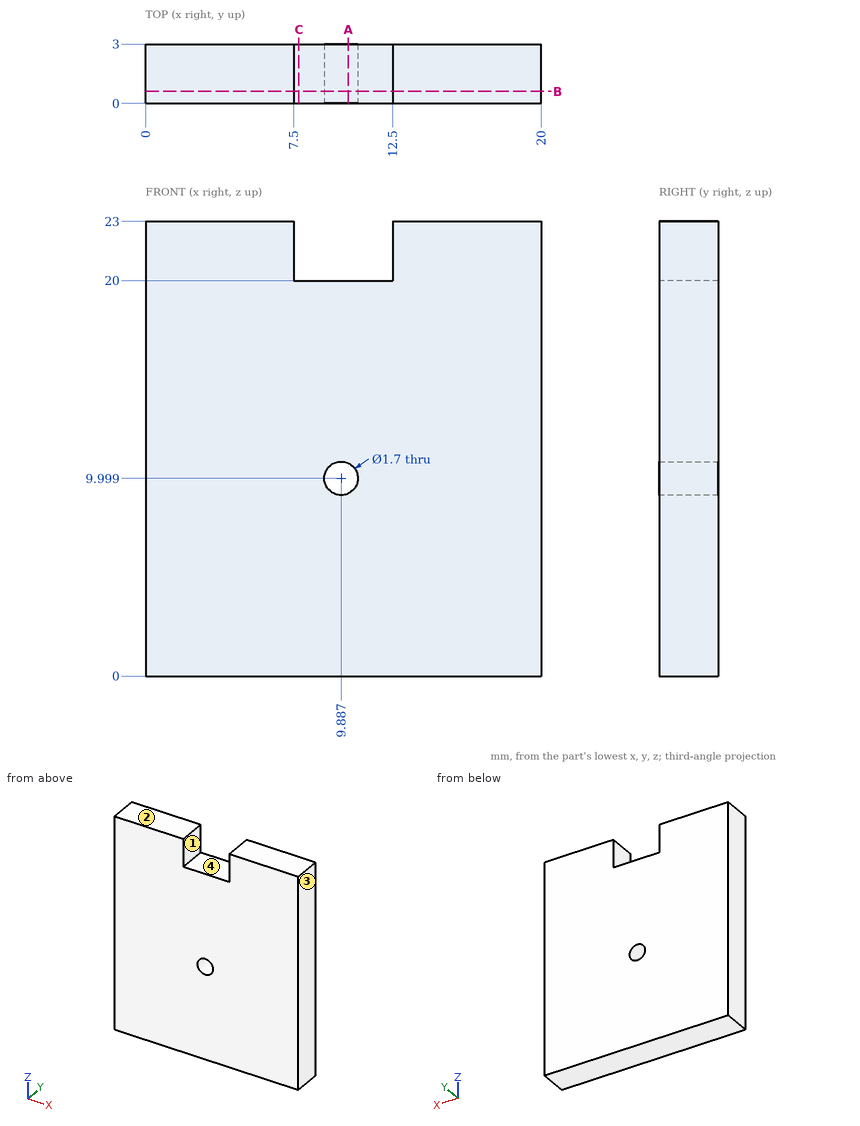
Drawing for the job (mm, zero at the part's lowest x, y, z). Give positions to 0.01 mm unless a question says otherwise; leave off trailing zeros. Order: outer loops, then holes, each group sorted by start corner. A loop starts at its lowest first (then second) coordinate and runs counter-clockwise, first axis right, second up. Notation, with made-up numbers: (-25.75, 61.5) - (31.25, 61.5) arc R16 ccw to (31.25, 83.5) - close; hole circle Ø4 at (29, -10.75). An arc over 180 degrees is marked (long way). Use one line per item in the form item = value.
Item 1: Slice it at B-B on y = 0.6. Give the cut face in (x, z).
Solution:
outline = (0, 0) - (20, 0) - (20, 23) - (12.5, 23) - (12.5, 20) - (7.5, 20) - (7.5, 23) - (0, 23) - close; hole circle Ø1.7 at (9.89, 10)
Item 2: Pin check, flat tips, straight feed: pin 1 Ø1 at (x, z) = (9.89, 10) entering from +Y; pin 2 Ø1.5 at (x, y) = (9, 1.5) entering from +Z. Stop position of each tip, or through.
Solution:
pin_1 = through
pin_2 = 20
Item 3: Slice it at A-A on x = 10.25. Give the cut face in (y, z).
Solution:
outline = (0, 0) - (3, 0) - (3, 9.23) - (0, 9.23) - close; (0, 10.77) - (3, 10.77) - (3, 20) - (0, 20) - close
Item 4: Probe probe 1 along X at (y, z) = (2.85, 10); probe 2 along Z at (x, y) = (9, 1.5). List the from-to ranges inside material, lowest first. Write a range as from..to.
Solution:
probe_1 = 0..9.04, 10.74..20
probe_2 = 0..20
Item 5: Slice it at C-C on x = 7.75. Give the cut face in (y, z), and give its area (3 significant figures).
Solution:
outline = (0, 0) - (3, 0) - (3, 20) - (0, 20) - close
area = 60.0 mm2
Item 6: Two-plate mould, pull along X, no slides. Class the marked faces 1, 2, 3 and 4: released by +X, released by -X, zero draft, split by the parting line, or undercut.
Solution:
face_1 = undercut
face_2 = zero draft
face_3 = released by +X
face_4 = undercut
